Print and shaded views of the part. All mm, measured from the part's lowest x, y and z. A direction names the side the tool comes from. Coordinates: 2 decimals unless noted, no trailing zeros. Order: outer loops, then holes, each group sorted by start corner. A loop starts at its lowest first (then second) coordinate and runs counter-clockwise, first axis right, second up. Notation, with made-up numbers: (79, 16) - (113, 16) arc R27 ccw to (113, 37) - close; hole circle Ø3 at (17, 88). An arc over 180 degrees is marked (long way). Write each question's results on one line, items separated by ' | '.
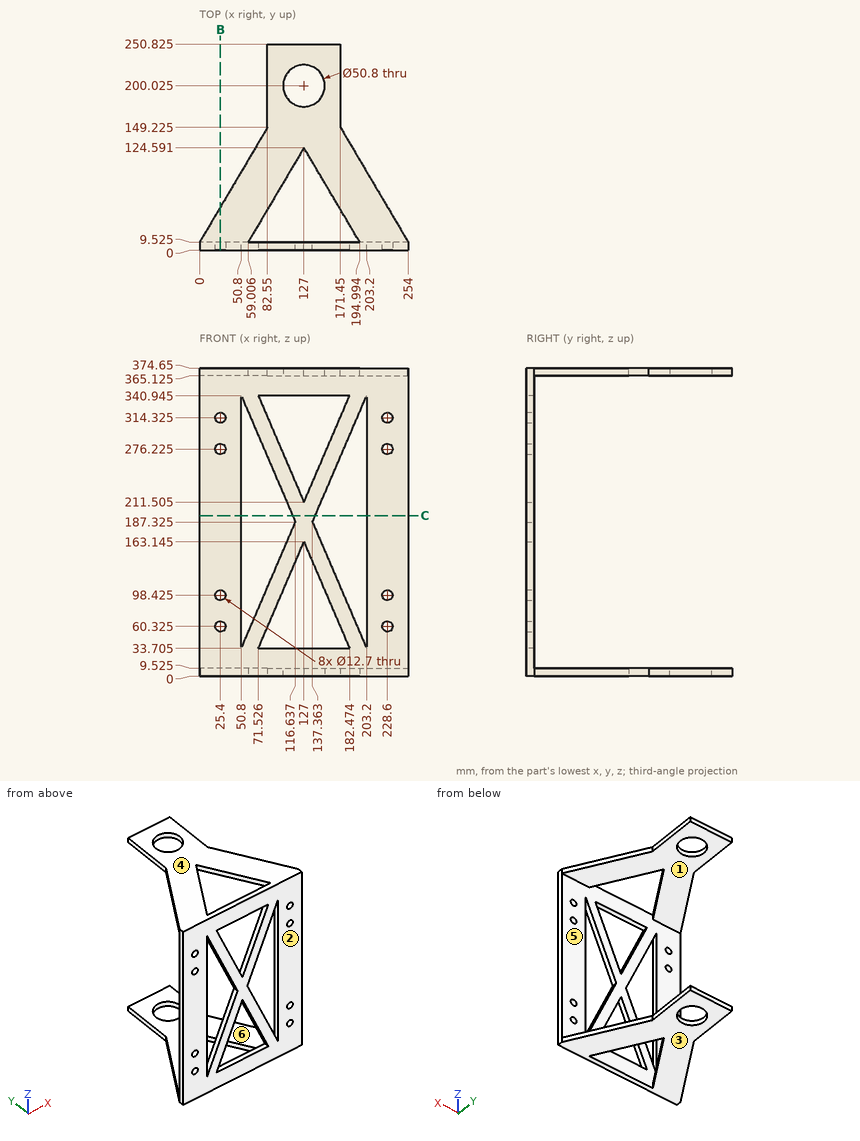
1. Band-saw the part on B-B on x = 25.4. Give the number of separate pieces and of enclosed holes in the cut face, then the cut area to 3 significant figures.
Solved:
separate pieces: 5 | enclosed holes: 0 | area: 3,900 mm2
2. Band-saw the part on C-C on z = 195. Give the cut face in (x, y) (1 decimal), then the cut area to 3 significant figures.
Solved:
outline: (0, 0) - (50.8, 0) - (50.8, 9.5) - (0, 9.5) - close; (113.3, 0) - (140.7, 0) - (140.7, 9.5) - (113.3, 9.5) - close; (203.2, 0) - (254, 0) - (254, 9.5) - (203.2, 9.5) - close | area: 1,230 mm2
3. Two-plate mould, pull along Z, no slides. Class the marked faces 3, 4, 5 and 6: +Z half, -Z half, draft (parallel to the pull), parting line (faces both ways), or undercut.
Solved:
face 3: -Z half | face 4: +Z half | face 5: undercut | face 6: undercut
4. Probe line 1 (Z direction, x = 228, y = 5); line 2 (Z direction, x = 25, y = 3); line 3 (Y direction, x = 173, z = 310) (1 decimal). List the from-to ranges inside material, lowest first.
Solved:
line 1: z = 0 to 54, 66.65 to 92.1, 104.75 to 269.9, 282.55 to 308, 320.65 to 374.65 | line 2: z = 0 to 53.99, 66.66 to 92.09, 104.76 to 269.89, 282.56 to 307.99, 320.66 to 374.65 | line 3: y = 0 to 9.5
5. Drop flat-ended pins along their axis: pin 1 Ø7.5 at (x, z) = (25.4, 276.225) entering from +Y; pin 2 Ø7.5 at (y, z) = (221, 369.5) entering from -X; pin 3 Ø3 at (y, z) = (218, 371) entering from +X; pin 4 Ø14.5 at (x, z) = (25.4, 60.325) entering from +Y (3 decimals). Give the stop position or say it passes through.
Solved:
pin 1: passes through | pin 2: stops at x = 82.55 | pin 3: stops at x = 171.45 | pin 4: stops at y = 9.525
6. Tool access for the marked faces 1 and 2: list every direction of +Z, -Z, +X, -X, +Y, -Y with a clear straight run to the whole face (end or side of a thin tool).
Solved:
face 1: +X, -X, +Y | face 2: +Z, -Z, +X, -X, -Y
